```python
from build123d import *

# Parameters (mm, degrees)
F0_R     = 97
F1_DEPTH = 5
F3_R     = 102
F3_R_2   = 97
F4_DEPTH = 5
F5_R     = 1.5
F6_R     = 4.99999
F2_R     = 2.5
F7_DEPTH = 5


# Not quite as in the source:
# - a fillet or chamfer is up to 0.001 mm smaller than in the source, because OpenCascade refuses the exact size


with BuildPart() as f1:
    # F0 (on Top) → F1 (new body)
    with BuildSketch(Plane.XY):
        with BuildLine():
            Line((-90, -110), (90, -110))
            ThreePointArc((90, -110), (104.1421356237, -104.1421356237), (110, -90))
            Line((110, -90), (110, 90))
            ThreePointArc((110, 90), (104.1421356237, 104.1421356237), (90, 110))
            Line((90, 110), (-90, 110))
            ThreePointArc((-90, 110), (-104.1421356237, 104.1421356237), (-110, 90))
            Line((-110, 90), (-110, -90))
            ThreePointArc((-110, -90), (-104.1421356237, -104.1421356237), (-90, -110))
        make_face()
        Circle(F0_R, mode=Mode.SUBTRACT)
    extrude(amount=F1_DEPTH)

    # F3 (on face) → F4 (join)
    with BuildSketch(Plane(origin=(0, 0, 0), x_dir=(1, 0, 0), z_dir=(0, 0, -1))):
        Circle(F3_R)
        Circle(F3_R_2, mode=Mode.SUBTRACT)
    extrude(amount=F4_DEPTH)

    # F5
    f5_edges = [f1.edges().sort_by_distance(p)[0] for p in [
        (-97, 0, -5),
        (-102, 0, -5),
        (-97, 0, 5),
    ]]
    fillet(f5_edges, radius=F5_R)

    # F6 (radius 5 in the source; OpenCascade refuses exactly that, so slightly less here)
    f6_edges = [f1.edges().sort_by_distance(p)[0] for p in [
        (-98.5, 0, 5),
        (0, -110, 5),
        (104.142136, -104.142136, 5),
        (110, 0, 5),
        (104.142136, 104.142136, 5),
        (0, 110, 5),
        (-104.142136, 104.142136, 5),
        (-110, 0, 5),
        (-104.142136, -104.142136, 5),
    ]]
    fillet(f6_edges, radius=F6_R)

    # F2 (on face) → F7 (cut, through all)
    with BuildSketch(Plane(origin=(0, 0, 0), x_dir=(1, 0, 0), z_dir=(0, 0, -1))):
        with Locations((-77, 77)):
            Circle(F2_R)
        with Locations((77, 77)):
            Circle(F2_R)
        with Locations((77, -77)):
            Circle(F2_R)
        with Locations((-77, -77)):
            Circle(F2_R)
    extrude(amount=-F7_DEPTH, mode=Mode.SUBTRACT)


solid = f1.part
```
For this review, take the finished solid that the model builds, in its own axes (mm). A direction names the side the tool comes from. Round coordinates to 2 decimals unless told otherwise and drop trailing zeros. One line per item, written item: value. Start each with the question number.
(1) Machinability: for faces 1 (the flat face through (48.4, 90.1, 0)), 2 (the cylindrical face through (1, -109, 3)), which of the approach directions +Z, -Z, +X, -X, +Y, -Y give a long, thin tool a straight path to every point of the face, cutting with its end or side? Answer none if there is none.
(2) Insertion check: pin 1 (1.5 mm diameter, centred on y = -51.5, z = -2, fed in from +X); pin 2 (1 mm diameter, centred on x = -12, z = 2, fed in from -Y); pin 3 (10 mm diameter, centred on x = -71.5, y = -87.5, fed in from -Z). Each pin has a flat end and moves straight along its axis. Give the tip position at first contact, or say it passes through.
(3) We need section C-C (x = -77). Count the separate pieces of the cut face and the enclosed holes in it, and give its area (3 significant figures).
(4) Wall thickness on line 1 (Y direction, x = -77, z = 2.95); line 2 (X direction, y = -79, z = 4); line 3 (X direction, y = 77, z = 3.9): over which ranges is each line inside the solid? List them lowest first.
(5) The part is to be moulded in two halves that separate along X. For faces 3 (the cylindrical face through (-109, -1, 3)), 4 (the cylindrical face through (-22.112, 99.574, -1.726)), 5 (the flat face through (-32, 94, 5)), 6 (the cylindrical face through (74.5, -77.1, 2.5)), say which applies: released by +X, released by -X, zero draft, split by the parting line, or undercut.
Result:
1. face 1: -Z
1. face 2: +Z, +X, -X, -Y
2. pin 1: x = 88.48
2. pin 2: y = -109.77
2. pin 3: z = 0
3. separate pieces: 4
3. enclosed holes: 0
3. area: 524 mm²
4. line 1: -109.04 to -79.5, -74.5 to -58.99, 58.99 to 74.5, 79.5 to 109.04
4. line 2: -108 to -78.5, -75.5 to -56.43, 56.43 to 75.5, 78.5 to 108
4. line 3: -108.13 to -79.5, -74.5 to -59.08, 59.08 to 74.5, 79.5 to 108.13
5. face 3: released by -X
5. face 4: split by the parting line
5. face 5: zero draft
5. face 6: undercut
